Input: dimensioned drawing with shaded views. Units: mm. Origin: part minimum x, y, z. Give positions to 0.01 mm unless a question says otherwise; leave off trailing zeros. Loops run counter-clockwise (first coordinate to the right, second up) from the corner with the lowest first, then second, coordinate; pieces in that order, holes last.
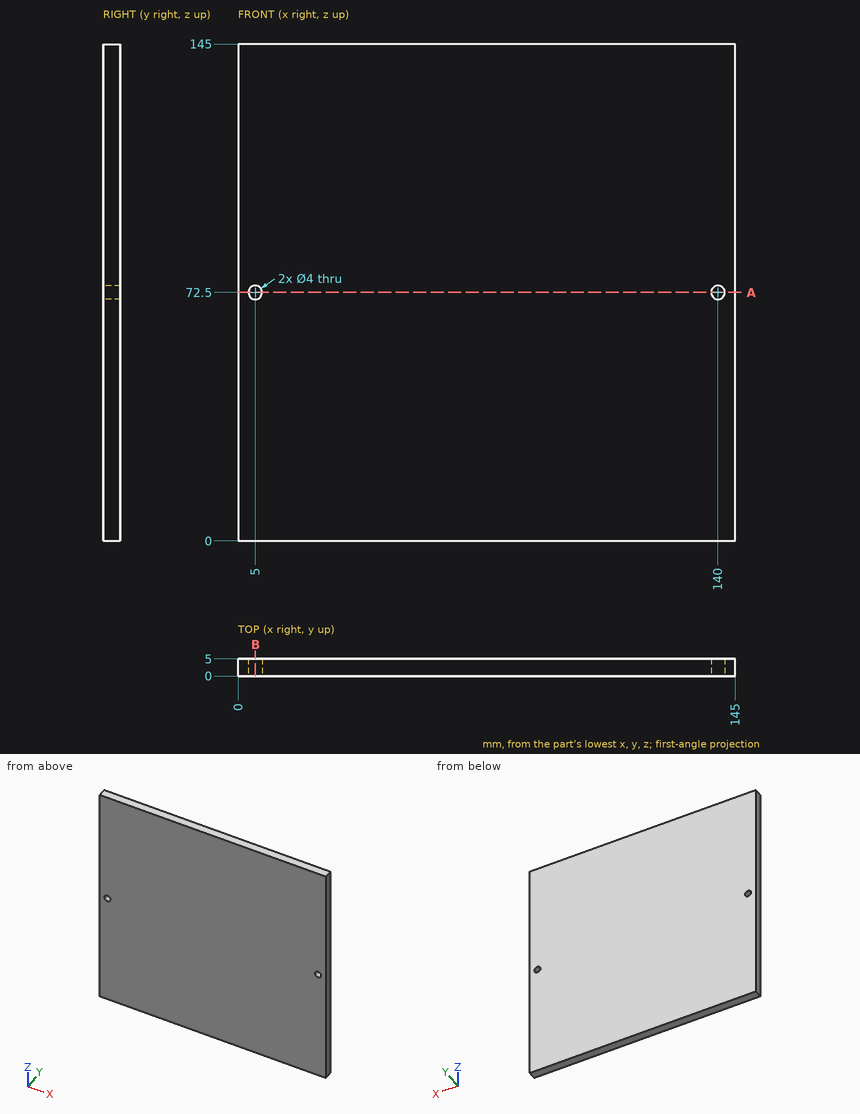
Item 1: Section query A-A on z = 72.5. Return loops of the section in (x, y), plus the area to 3 significant figures.
Values follow:
outline: (0, 0) - (3, 0) - (3, 5) - (0, 5) - close; (7, 0) - (138, 0) - (138, 5) - (7, 5) - close; (142, 0) - (145, 0) - (145, 5) - (142, 5) - close
area: 685 mm2
Item 2: Ray query, probe 1 along X at (y, z) = (1.7, 72.5); probe 2 along Z at (x, y) = (5, 1.1). Return the intervals inside material, ascending.
Values follow:
probe 1: x = 0 to 3, 7 to 138, 142 to 145
probe 2: z = 0 to 70.5, 74.5 to 145
Item 3: Section query B-B on x = 5. Return loops of the section in (y, z), plus the area to 3 significant figures.
Values follow:
outline: (0, 0) - (5, 0) - (5, 70.5) - (0, 70.5) - close; (0, 74.5) - (5, 74.5) - (5, 145) - (0, 145) - close
area: 705 mm2
